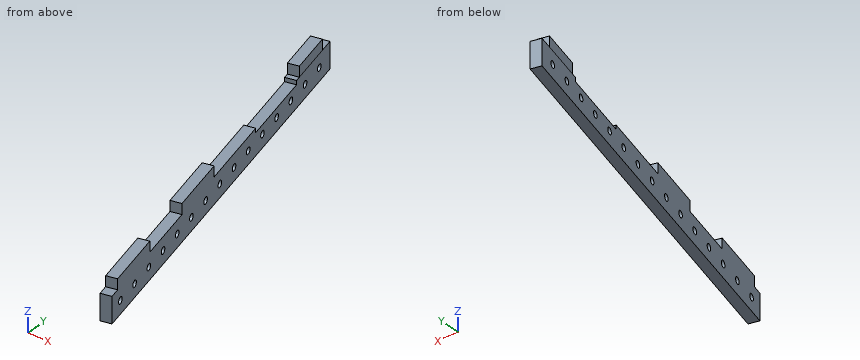
from build123d import *

# Parameters (mm, degrees)
BOSS_EXTRUDE1_DEPTH   = 10.16
BOSS_EXTRUDE1_2_DEPTH = 10.16
BOSS_EXTRUDE1_3_DEPTH = 10.16
BOSS_EXTRUDE2_DEPTH   = 25.4
SKETCH3_R             = 3.175
SKETCH3_W             = 29.218678694
SKETCH3_H             = 73
CUT_EXTRUDE1_DEPTH    = 1837.667023453


with BuildPart() as part:
    # Sketch1 → Boss-Extrude1 (new body)
    with BuildSketch(Plane.XY):
        Polygon((-120.524654614, 1641.945974367), (-107.584015199, 1585.893906943), (-117.483615058, 1583.608404231), (-130.424254473, 1639.660471655), align=None)
    extrude(amount=-BOSS_EXTRUDE1_DEPTH)



with BuildPart() as body_2:
    # Sketch1 → Boss-Extrude1 2 (new body)
    with BuildSketch(Plane.XY):
        Polygon((-104.542975642, 1527.556336807), (-94.643375784, 1529.841839519), (-81.702736369, 1473.789772095), (-91.602336227, 1471.504269383), align=None)
    extrude(amount=-BOSS_EXTRUDE1_2_DEPTH)


with BuildPart() as body_3:
    # Sketch1 → Boss-Extrude1 3 (new body)
    with BuildSketch(Plane.XY):
        Polygon((-164.706795155, 1788.154469528), (-154.807195296, 1790.43997224), (-164.092050064, 1830.657096664), (-173.991649923, 1828.371593952), align=None)
    extrude(amount=-BOSS_EXTRUDE1_3_DEPTH)


with BuildPart() as part_1:
    add(part.part)

    add(body_2.part)  # Boss-Extrude2 merges body 2

    add(body_3.part)  # Boss-Extrude2 merges body 3
    # Sketch2 → Boss-Extrude2 (add)
    with BuildSketch(Plane(origin=(0, 0, -10.16), x_dir=(-1, 0, 0), z_dir=(0, 0, -1))):
        Polygon((177.016251562, 1841.472582982), (89.352825684, 1461.760568735), (79.453225826, 1464.046071447), (167.116651704, 1843.758085694), align=None)
    extrude(amount=BOSS_EXTRUDE2_DEPTH)

    # Sketch3 → Cut-Extrude1 (cut, through all)
    with BuildSketch(Plane(origin=(235.565521709, 54.384585889, 0), x_dir=(0, 0, 1), z_dir=(-0.974370064785235, -0.22495105434386642, 0))):
        with Locations(Location((-22.86, 1459.395752405, 0), (0, 0, 270))):
            Circle(SKETCH3_R)
        with Locations(Location((-22.86, 1484.795752405, 0), (0, 0, 270))):
            Circle(SKETCH3_R)
        with Locations(Location((-22.86, 1510.195752405, 0), (0, 0, 270))):
            Circle(SKETCH3_R)
        with Locations(Location((-22.86, 1535.595752405, 0), (0, 0, 270))):
            Circle(SKETCH3_R)
        with Locations(Location((-22.86, 1560.995752405, 0), (0, 0, 270))):
            Circle(SKETCH3_R)
        with Locations(Location((-22.86, 1586.395752405, 0), (0, 0, 270))):
            Circle(SKETCH3_R)
        with Locations(Location((-22.86, 1611.795752405, 0), (0, 0, 270))):
            Circle(SKETCH3_R)
        with Locations(Location((-22.86, 1637.195752405, 0), (0, 0, 270))):
            Circle(SKETCH3_R)
        with Locations(Location((-22.86, 1662.595752405, 0), (0, 0, 270))):
            Circle(SKETCH3_R)
        with Locations(Location((-22.86, 1687.995752405, 0), (0, 0, 270))):
            Circle(SKETCH3_R)
        with Locations(Location((-22.86, 1713.395752405, 0), (0, 0, 270))):
            Circle(SKETCH3_R)
        with Locations(Location((-22.86, 1738.795752405, 0), (0, 0, 270))):
            Circle(SKETCH3_R)
        with Locations(Location((-22.86, 1764.195752405, 0), (0, 0, 270))):
            Circle(SKETCH3_R)
        with Locations(Location((-22.86, 1789.595752405, 0), (0, 0, 270))):
            Circle(SKETCH3_R)
        with Locations(Location((-22.86, 1814.995752405, 0), (0, 0, 270))):
            Circle(SKETCH3_R)
        with Locations((0.449339347, 1737.875153548)):
            Rectangle(SKETCH3_W, SKETCH3_H)
    extrude(amount=-CUT_EXTRUDE1_DEPTH, mode=Mode.SUBTRACT)


solid = part_1.part
CAD build for the part. Positions are in the model's coordinates, mm. Coordinates: 2 decimals unless noted, no trailing zeros. Loops run counter-clockwise (first coordinate to the right, second up) from the corner with the lowest first, then second, coordinate; pieces in that order, holes last. Notation, with made-up numbers: (55, -13) - (101, -13) arc R35 ccw to (101, 23) - close; hole circle Ø7 at (25.5, 43). An arc over 180 degrees is marked (long way). Use one line per item in the form item = value. Start each with the question number.
1) Flat gauge pins, fed straight in: pin 1 (18.5 mm diameter, centred on x = -108, y = 1569, fed in from +Z); pin 2 (13 mm diameter, centred on x = -88, y = 1466, fed in from +Z); pin 3 (1.5 mm diameter, centred on y = 1773.5, z = -14.5, fed in from -X); pin 4 (13 mm diameter, centred on x = -155, y = 1760, fed in from +Z). Where does each tip first touch, or does it go through?
2) Band-saw the part on A-A (z = -3.5). Give the cut face in (x, y).
3) Band-saw the part on B-B (y = 1542). Give the cut face in (x, z), and give its area (3 significant figures).
4) Band-saw the part on C-C (y = 1758). Give the cut face in (x, z).
5) Drill centre lines: L1, parallel to Z at x = -109, y = 1548; L2, parallel to X at y = 1641.5, z = -32; L3, parallel to X at y = 1532, z = -23. Where is each one in solid material? Low to high. Write a range as from..to.
Check values:
q1.pin_1 = -10.16
q1.pin_2 = 0
q1.pin_3 = -161.5
q1.pin_4 = -14.16
q2.outline = (-173.99, 1828.37) - (-164.71, 1788.15) - (-154.81, 1790.44) - (-164.09, 1830.66) - close; (-130.42, 1639.66) - (-117.48, 1583.61) - (-107.58, 1585.89) - (-120.52, 1641.95) - close; (-104.54, 1527.56) - (-91.6, 1471.5) - (-81.7, 1473.79) - (-94.64, 1529.84) - close
q3.outline = (-107.88, -35.56) - (-97.45, -35.56) - (-97.45, -10.16) - (-107.88, -10.16) - close
q3.area = 265 mm2
q4.outline = (-157.75, -35.56) - (-147.32, -35.56) - (-147.32, -14.16) - (-157.75, -14.16) - close
q5.L1 = -35.56..-24.44, -21.28..-10.16
q5.L2 = -130.85..-120.42
q5.L3 = -105.57..-95.14
